Autodesk Fusion 360 part; units mm, degrees
sketch "Sketch1" plane through (0, 0, 0) normal (0, 0, 1) x (1, 0, 0)
  circle A0 centre (0, 0) radius 10
  line L0 (-1.778, 1.778) -> (1.778, 1.778)
  line L1 (1.778, 1.778) -> (1.778, -1.778)
  line L2 (1.778, -1.778) -> (-1.778, -1.778)
  line L3 (-1.778, -1.778) -> (-1.778, 1.778)
  line L4 (-1.778, 1.778) -> (1.778, -1.778) construction
  line L5 (1.778, 1.778) -> (-1.778, -1.778) construction
  line L6 (0, 10) -> (0, -50.96)
  line L7 (0, -50.96) -> (11.2783, -42.9344)
  line L8 (0, -50.96) -> (6.4922, -31.3521)
  line L9 (9.8281, 1.8461) -> (16.0511, -31.2832)
  line L10 (11.2783, -42.9344) -> (16.0511, -31.2832)
  line L11 (6.4922, -31.3521) -> (0, -10)
  point P0 (-10, 0)
  point P1 (0, 10)
  dimension "d1" = 20
  dimension "d5" = 3.556
  dimension "d14" = 60.96
extrude "Extrude1" add sketch "Sketch1" along normal blind 6 contours A0 L0 L1 L2 L6 | A0 L7 L8 L9 L10 L11 | A0 L0 L2 L3 L6
fillet "Fillet5" radius 24.5 2 edges at (16.0511, -31.2832, 3) (11.2783, -42.9344, 3)
fillet "Fillet6" radius 0.5 1 edges at (0, -50.96, 3)
fillet "Fillet7" radius 20 1 edges at (6.4922, -31.3521, 3)
fillet "Fillet8" radius 5.5 1 edges at (0, -10, 3)
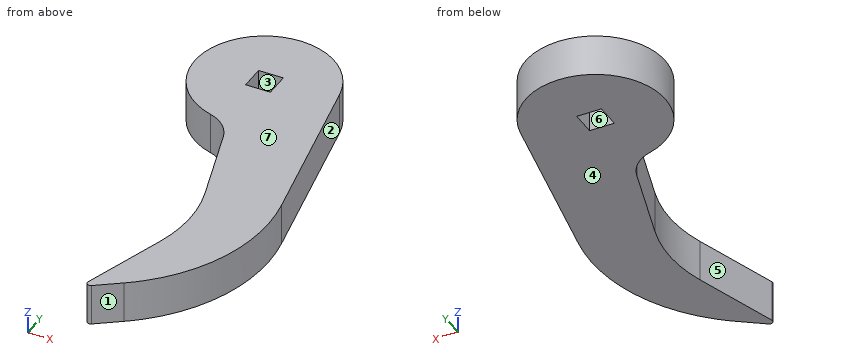
Read the model definition and answer for the solid it produces. Units are mm, in the model's axes. Face numbers are marked on the shaded views. A direction names the side the tool comes from. Give positions to 0.01 mm unless a question says otherwise; leave off trailing zeros. Write each loop counter-clockwise with the first axis right and the second up, starting at its lowest first coordinate (ties: lowest second). Pieces come first, ordered by that corner, then holes. Notation, with made-up numbers: (-17, 45) -> (6, 45) arc R10 cw to (6, 50) -> close; hole circle Ø10 at (81.25, 8). An arc over 180 degrees is marked (long way). Answer in a Markdown table with one row per item.
1) Each of these flat-tipped pins is pushed along its axis until it touches: pin 1 Ø1.5 at (y, z) = (-14.5, 2) entering from +X; pin 2 Ø1 at (y, z) = (-32, 1.5) entering from -X; pin 3 Ø3 at (y, z) = (-23, 4) entering from +X. Where does it stop, or does it pass through?
Results list:
| item | result |
|---|---|
| pin 1 | x = 13.04 |
| pin 2 | x = 5.46 |
| pin 3 | x = 14.74 |
2) Section A-A on y = 0 is taken. Give the vertices of the cut face in (x, z).
Results list:
| item | result |
|---|---|
| outline | (-10, 0) -> (-1.78, 0) -> (-1.78, 6) -> (-10, 6) -> close; (1.78, 0) -> (10.17, 0) -> (10.17, 6) -> (1.78, 6) -> close |
3) Determine the mould class of the marked faces 1, 2, 3 and 4 for opening direction Y: released by +Y, released by -Y, zero draft, split by the parting line, or undercut.
Results list:
| item | result |
|---|---|
| face 1 | released by -Y |
| face 2 | released by +Y |
| face 3 | undercut |
| face 4 | zero draft |
4) A tool of negligible diameter and unlimited length cuts with its end or side. For the marked faces 5, 6 and 7, from which of +Z, -Z, +X, -X, +Y, -Y can it reach the whole face along a straight path? Write none if from no direction.
Results list:
| item | result |
|---|---|
| face 5 | +Z, -Z, -X |
| face 6 | +Z, -Z |
| face 7 | +Z, +X, -X, +Y, -Y |
5) Section C-C on y = -16 is taken. Give the vertices of the cut face in (x, z).
Results list:
| item | result |
|---|---|
| outline | (1.82, 0) -> (13.18, 0) -> (13.18, 6) -> (1.82, 6) -> close |
6) Straight lines are drawn through the part: line 1 (X direction, y = 1, z = 4.25); line 2 (Y direction, x = -1.25, z = 1); line 3 (Y direction, x = -1.5, z = 2). For each, find the intervals that lie inside material, in ascending order. Write a range as [from, to].
Results list:
| item | result |
|---|---|
| line 1 | [-9.95, -1.78], [1.78, 9.99] |
| line 2 | [-10.3, -1.78], [1.78, 9.92] |
| line 3 | [-10.15, -1.78], [1.78, 9.89] |
7) Section B-B on x = -8 is taken. Give the vertices of the cut face in (y, z), plus the area to 3 significant figures.
Results list:
| item | result |
|---|---|
| outline | (-6, 0) -> (6, 0) -> (6, 6) -> (-6, 6) -> close |
| area | 72.0 mm^2 |
